from build123d import *

# Parameters (mm, degrees)
F0_W     = 14.9271550402
F0_H     = 6
F1_DEPTH = 1
F2_R     = 0.25
F3_DEPTH = 1
F0_W_2   = 6
F0_H_2   = 12
F4_DEPTH = 1
F5_R     = 0.5


# Not quite as in the source:
# - a feature names something its author has since deleted; it is built from what else it names


with BuildPart() as f1:
    # F0 (on Top) → F1 (new body)
    with BuildSketch(Plane.XY):
        with Locations((-0.0364224799, 10.5)):
            Rectangle(F0_W, F0_H)
        Polygon((7.4271550402, 7.5), (-7.5, 7.5), (-7.5, -7.5), (7.4271550402, -7.5), (7.5, -7.5), (7.5, -6.1350027099), (7.5, 5.8649972901), (7.5, 7.5), align=None)
        with BuildLine():
            ThreePointArc((-5, 0), (-4.267766953, 1.767766953), (-2.5, 2.5))
            Line((-2.5, 2.5), (2.5, 2.5))
            ThreePointArc((2.5, 2.5), (4.267766953, 1.767766953), (5, 0))
            ThreePointArc((5, 0), (4.267766953, -1.767766953), (2.5, -2.5))
            Line((2.5, -2.5), (-2.5, -2.5))
            ThreePointArc((-2.5, -2.5), (-4.267766953, -1.767766953), (-5, 0))
        make_face(mode=Mode.SUBTRACT)
        with Locations((-0.0364224799, -10.5)):
            Rectangle(F0_W, F0_H)
    extrude(amount=F1_DEPTH)

    # F2
    f2_edges = [f1.edges().sort_by_distance(p)[0] for p in [
        (-0.036422, 13.5, 0),
        (-7.5, 0, 0),
        (-0.036422, -13.5, 0),
        (7.427155, -10.5, 0),
        (7.463578, -7.5, 0),
        (7.5, 0, 0),
        (7.463578, 7.5, 0),
        (7.427155, 10.5, 0),
        (-5, 0, 0),
        (0, 2.5, 0),
        (5, 0, 0),
        (0, -2.5, 0),
    ]]
    fillet(f2_edges, radius=F2_R)

    # F0 (on Top) → F3 (cut)
    with BuildSketch(Plane.XY):
        with BuildLine():
            Line((2.5, 2.5), (-2.5, 2.5))
            ThreePointArc((-2.5, 2.5), (-4.267766953, 1.767766953), (-5, 0))
            ThreePointArc((-5, 0), (-4.267766953, -1.767766953), (-2.5, -2.5))
            Line((-2.5, -2.5), (2.5, -2.5))
            ThreePointArc((2.5, -2.5), (4.267766953, -1.767766953), (5, 0))
            ThreePointArc((5, 0), (4.267766953, 1.767766953), (2.5, 2.5))
        make_face()
    extrude(amount=F3_DEPTH, mode=Mode.SUBTRACT)

    # F0 (on Top) → F4 (join)
    with BuildSketch(Plane.XY):
        with Locations((10.5, -0.1350027099)):
            Rectangle(F0_W_2, F0_H_2)
    extrude(amount=F4_DEPTH)

    # F5
    f5_edges = [f1.edges().sort_by_distance(p)[0] for p in [
        (-0.036422, 13.5, 1),
        (-7.5, 0, 1),
        (-0.036422, -13.5, 1),
        (7.427155, -10.5, 1),
        (7.463578, -7.5, 1),
        (7.5, -6.817501, 1),
        (10.5, -6.135003, 1),
        (13.5, -0.135003, 1),
        (10.5, 5.864997, 1),
        (7.5, 6.682499, 1),
        (7.463578, 7.5, 1),
        (7.427155, 10.5, 1),
        (-5, 0, 1),
        (0, 2.5, 1),
        (5, 0, 1),
        (0, -2.5, 1),
    ]]
    fillet(f5_edges, radius=F5_R)


solid = f1.part
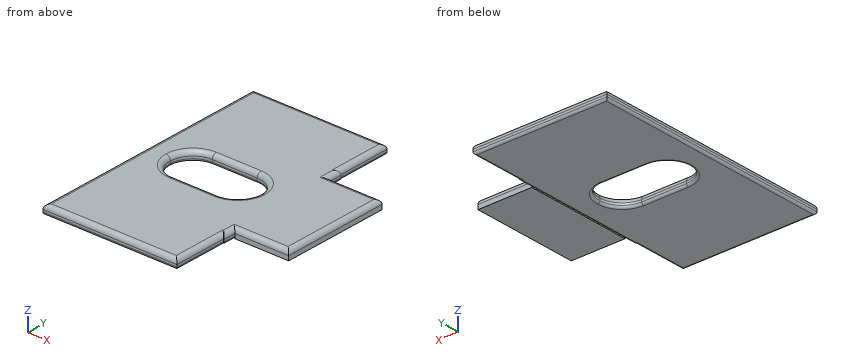
Here's how the part is built. I have some questions about the finished solid (model axes, mm). Give positions to 0.01 mm unless a question says otherwise; leave off trailing zeros. Order: outer loops, then holes, each group sorted by start corner. A loop starts at its lowest first (then second) coordinate and runs counter-clockwise, first axis right, second up. Notation, with made-up numbers: (7.25, 50) -> (60.25, 50) arc R19 cw to (60.25, 74) -> close; hole circle Ø7 at (-12.5, -13.5). An arc over 180 degrees is marked (long way). Use a Markdown table: item, result. Add a question column.
Item 1: Imagine slicing it at C-C on z = 0.85. Please give me the cut outline in (x, y).
Item 2: Imagine slicing it at A-A on x = -2. Please give me the cut outline in (y, z).
Item 3: Imagine slicing it at B-B on y = 8. Please give me the cut outline in (x, z).
Item 4: I need wall thicknesses on line 1 (Y direction, x = -0.5, z = 0.3); line 2 (Y direction, x = 8.5, z = 0.55); line 3 (Y direction, x = -3, z = 0.35). Which ranges of each line are inside material? Lowest first, please.
Item 5: Imagine slicing it at D-D on x = 10.5. Please give me the cut outline in (y, z) (3 decimals).
Data:
| question | item | result |
|---|---|---|
| 1 | outline | (-7.36, -13.36) -> (7.28, -13.36) -> (7.28, -7.36) -> (7.36, -7.36) -> (7.36, -5.99) -> (13.36, -5.99) -> (13.36, 5.72) -> (7.36, 5.72) -> (7.36, 7.36) -> (7.28, 7.36) -> (7.28, 13.36) -> (-7.36, 13.36) -> close; hole (-2.5, -2.64) -> (2.5, -2.64) arc R2.64 ccw to (2.5, 2.64) -> (-2.5, 2.64) arc R2.64 ccw to start |
| 2 | outline | (-13.5, 0.25) arc R0.25 ccw to (-13.25, 0) -> (-2.75, 0) arc R0.25 ccw to (-2.5, 0.25) -> (-2.5, 0.5) arc R0.5 ccw to (-3, 1) -> (-13, 1) arc R0.5 ccw to (-13.5, 0.5) -> close; (2.5, 0.25) arc R0.25 ccw to (2.75, 0) -> (13.25, 0) arc R0.25 ccw to (13.5, 0.25) -> (13.5, 0.5) arc R0.5 ccw to (13, 1) -> (3, 1) arc R0.5 ccw to (2.5, 0.5) -> close |
| 3 | outline | (-7.5, 0.25) arc R0.25 ccw to (-7.25, 0) -> (7.18, 0) arc R0.25 ccw to (7.43, 0.25) -> (7.43, 0.5) arc R0.5 ccw to (6.93, 1) -> (-7, 1) arc R0.5 ccw to (-7.5, 0.5) -> close |
| 4 | line 1 | y = -13.5 to -2.5, 2.5 to 13.5 |
| 4 | line 2 | y = -6.13 to 5.86 |
| 4 | line 3 | y = -13.5 to -2.45, 2.45 to 13.5 |
| 5 | outline | (-6.135, 0) -> (5.865, 0) -> (5.865, 0.5) arc R0.5 ccw to (5.365, 1) -> (-5.635, 1) arc R0.5 ccw to (-6.135, 0.5) -> close |
